```python
from build123d import *

# Parameters (mm, degrees)
F1_DEPTH = 76.2
F3_D     = 17.145
F3_DEPTH = 50.8
F3_TIP   = 5.1508776566
F5_D     = 12.7
F5_DEPTH = 50.8
F5_TIP   = 3.8154649308
F7_D     = 22.225


with BuildPart() as f1:
    # F0 (on Front) → F1 (new body)
    with BuildSketch(Plane.XZ):
        Polygon((-149.225, 0), (0, 0), (0, 50.8), (-76.2, 50.8), (-76.2, 101.6), (0, 101.6), (0, 152.4), (-149.225, 152.4), align=None)
        with BuildLine():
            ThreePointArc((-149.225, 152.4), (-225.425, 76.2), (-149.225, 0))
            Line((-149.225, 0), (-149.225, 152.4))
        make_face()
    extrude(amount=F1_DEPTH)

    # F3
    with Locations(Plane(origin=(0, 0, 0), x_dir=(1, 0, 0), z_dir=(0, 0, -1))):
        with Locations((-38.1, 38.1)):
            Hole(F3_D / 2, depth=F3_DEPTH)
            with Locations((0, 0, -(F3_DEPTH + F3_TIP / 2))):  # 118° drill point
                Cone(0, F3_D / 2, F3_TIP, mode=Mode.SUBTRACT)

    # F5
    with Locations(Plane.XY.offset(152.4)):
        with Locations((-38.1, -38.1)):
            Hole(F5_D / 2, depth=F5_DEPTH)
            with Locations((0, 0, -(F5_DEPTH + F5_TIP / 2))):  # 118° drill point
                Cone(0, F5_D / 2, F5_TIP, mode=Mode.SUBTRACT)

    # F7 (through all)
    with Locations(Plane(origin=(0, 0, 0), x_dir=(-1, 0, 0), z_dir=(0, 1, 0))):
        with Locations((114.3, 76.2)):
            Hole(F7_D / 2)


solid = f1.part
```
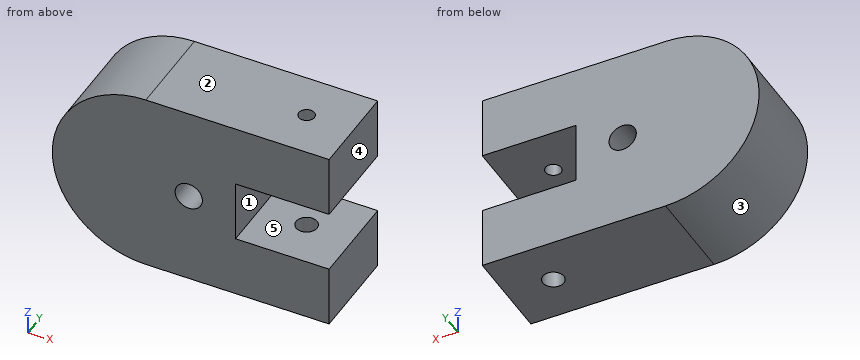
The listing builds one solid part. Answer for the finished solid, in the listing's coordinates (mm). Face numbers are marked on the shaded views. A direction names the side the tool comes from. Coordinates: 2 decimals unless noted, no trailing zeros. Loops run counter-clockwise (first coordinate to the right, second up) from the corner with the lowest first, then second, coordinate; pieces in that order, holes last. Notation, with made-up numbers: M -8.5,83 L 20.5,83 A14 ccw 20.5,98 Z; hole C 45,11 d4. An arc over 180 degrees is marked long. Answer as a JSON object with one key per item and string values. Group by question number.
Item 1: Which of the six approach directions +Z, -Z, +X, -X, +Y, -Y give full straight-line access (tool end or side, diameter ignored) to the marked faces 1 and 2?
Item 2: Consider L1, parallel to Z at x = -38.5, y = -50; L2, parallel to Y at x = -38, z = 33; L3, parallel to Z at x = -114.3, y = -20.5. Determine where each line is inside the solid, lowest interval first.
Item 3: Section A-A (y = -38.1) is taken. Give the number of separate pieces and of enclosed holes in the cut face, and give its area (3 significant figures).
Item 4: Section B-B (z = 76.2) is taken. Write down the section's boundary in (x, y) (1 decimal).
Item 5: Section C-C (x = -70.5) is taken. Write down the section's boundary in (y, z).
Item 6: Determine the mould class of the marked faces 3, 4 and 5 for opening direction Z: +Z half, -Z half, draft (parallel to the pull), parting line (faces both ways), or undercut.
Item 7: Section D-D (x = -38.1) is taken. Write down the section's boundary in (y, z).
Item 8: Each of these flat-tipped pins is pushed along its axis until it touches: P1, Ø12, axis at y = -59, z = 125.5, coming from the -X side; P2, Ø16.5, axis at x = -38.1, y = -38.1, coming from the +Z side; P3, Ø1.5, axis at y = -35.5, z = 39.5, coming from the -X side; P4, Ø1.5, axis at y = -44, z = 23.5, coming from the -X side. Where does it stop, or does it pass through?
Solved:
{
 "1": {"face 1": "+X, +Y, -Y", "face 2": "+Z, +X, -X, +Y, -Y"},
 "2": {"L1": "z = 0 to 50.8, 101.6 to 152.4", "L2": "y = -76.2 to -46.67, -29.53 to 0", "L3": "z = 0 to 65.09, 87.31 to 152.4"},
 "3": {"separate pieces": "3", "enclosed holes": "1", "area": "26,100 mm2"},
 "4": {"outline": "M -225.4,-76.2 L -125.4,-76.2 L -125.4,0 L -225.4,0 Z; M -103.2,-76.2 L -76.2,-76.2 L -76.2,0 L -103.2,0 Z"},
 "5": {"outline": "M -76.2,0 L 0,0 L 0,50.8 L -76.2,50.8 Z; M -76.2,101.6 L 0,101.6 L 0,152.4 L -76.2,152.4 Z"},
 "6": {"face 3": "parting line", "face 4": "draft", "face 5": "undercut"},
 "7": {"outline": "M -76.2,0 L -46.67,0 L -46.67,50.8 L -76.2,50.8 Z; M -76.2,101.6 L -44.45,101.6 L -44.45,152.4 L -76.2,152.4 Z; M -31.75,101.6 L 0,101.6 L 0,152.4 L -31.75,152.4 Z; M -29.53,0 L 0,0 L 0,50.8 L -29.53,50.8 Z"},
 "8": {"P1": "stops at x = -211.93", "P2": "stops at z = 152.4", "P3": "stops at x = -216.41", "P4": "stops at x = -204.97"}
}
